Part model, mm, in its own coordinate system. A direction names the side the tool comes from. Give positions to 0.01 mm unless a question says otherwise; leave off trailing zeros. Write each loop counter-clockwise with the first axis right and the second up, starting at its lowest first coordinate (ties: lowest second). Pieces come first, ordered by that corner, then holes. Notation, with made-up numbers: (43.5, -14) - (99.5, -14) arc R8 ccw to (99.5, 0) - close; hole circle Ø5 at (37.25, 81.5). An arc over 180 degrees is marked (long way). Answer in a Markdown table with one row per item. Add a question column.
1. Probe line 1 along Y through (x, z) = (0, 1); line 2 along Y through (x, z) = (-20, 0.8); line 3 along X through (y, z) = (1, 4.75). List the from-to ranges inside material, lowest first.
2. Pull direction Y, two halves, no side cores. Call faces 6 (the flat face through (10, -30, 1)), 7 (the flat face through (-17.7, -2.3, 2)), 8 (the flat face through (-19, -8, 5)): released by +Y, released by -Y, zero draft, split by the parting line, or undercut.
3. Which spindle directions (+Z, -Z, +X, -X, +Y, -Y) get a long thin tool onto all of the face, cutting with end or side? Do faces 1 (the flat face through (18, -8, 5)), 2 (the flat face through (-20, -10, 1)), 3 (the flat face through (0, -48, 5)), 4 (the cylindrical face through (14.755, 0.231, 4.028)), 5 (the flat face through (-8, -28, 5)). Say none if no direction does.
4. Band-saw the part on A-A on x = 0. State how many separate pieces and enclosed holes the cut face has, plus the area to 3 significant figures.
5. Drop flat-ended pins along their axis: pin 1 Ø13.5 at (x, y) = (20, 0) entering from -Z; pin 2 Ø2.5 at (y, z) = (-21, 1.5) entering from +X; pin 3 Ø3.5 at (x, z) = (-23.5, 1) entering from -Y; pin 4 Ø6.5 at (x, y) = (0, 0) entering from +Z. Give the stop position or say it passes through.
6. Band-saw the part on D-D on x = 20. Write the cut outline in (y, z).
7. Band-saw the part on B-B on z = 5. Write the cut outline in (x, y).
```python
from build123d import *

# Parameters (mm, degrees)
F2_R     = 2.75
F3_DEPTH = 6
F4_SIZE  = 3
F5_R     = 5.25
F5_R_2   = 2.75
F6_DEPTH = 4


with BuildPart() as f3:
    # F2 (on Top) → F3 (new body)
    with BuildSketch(Plane.XY):
        Polygon((-10, -50), (0, -50), (10, -50), (10, -10), (30, -10), (30, 10), (0, 10), (-30, 10), (-30, -10), (-10, -10), align=None)
        with Locations((0, -40)):
            Circle(F2_R, mode=Mode.SUBTRACT)
        with Locations((-20, 0)):
            Circle(F2_R, mode=Mode.SUBTRACT)
        with Locations((0, -20)):
            Circle(F2_R, mode=Mode.SUBTRACT)
        Circle(F2_R, mode=Mode.SUBTRACT)
        with Locations((20, 0)):
            Circle(F2_R, mode=Mode.SUBTRACT)
    extrude(amount=F3_DEPTH)

    # F4
    f4_edges = [f3.edges().sort_by_distance(p)[0] for p in [
        (0, -50, 6),
        (10, -30, 6),
        (20, -10, 6),
        (30, 0, 6),
        (0, 10, 6),
        (-30, 0, 6),
        (-20, -10, 6),
        (-10, -30, 6),
    ]]
    chamfer(f4_edges, length=F4_SIZE)

    # F5 (on face) → F6 (cut)
    with BuildSketch(Plane.XY.offset(6)):
        with Locations((-20, 0)):
            Circle(F5_R)
        with Locations((-20, 0)):
            Circle(F5_R_2, mode=Mode.SUBTRACT)
        Circle(F5_R)
        Circle(F5_R_2, mode=Mode.SUBTRACT)
        with Locations((20, 0)):
            Circle(F5_R)
        with Locations((20, 0)):
            Circle(F5_R_2, mode=Mode.SUBTRACT)
        with Locations((0, -20)):
            Circle(F5_R)
        with Locations((0, -20)):
            Circle(F5_R_2, mode=Mode.SUBTRACT)
        with Locations((0, -40)):
            Circle(F5_R)
        with Locations((0, -40)):
            Circle(F5_R_2, mode=Mode.SUBTRACT)
    extrude(amount=-F6_DEPTH, mode=Mode.SUBTRACT)


solid = f3.part
```
Values:
| question | item | result |
|---|---|---|
| 1 | line 1 | y = -50 to -42.75, -37.25 to -22.75, -17.25 to -2.75, 2.75 to 10 |
| 1 | line 2 | y = -10 to -2.75, 2.75 to 10 |
| 1 | line 3 | x = -28.25 to -25.15, -14.85 to -5.15, 5.15 to 14.85, 25.15 to 28.25 |
| 2 | face 6 | zero draft |
| 2 | face 7 | undercut |
| 2 | face 8 | released by -Y |
| 3 | face 1 | +Z, +X, -Y |
| 3 | face 2 | +Z, -Z, -X, -Y |
| 3 | face 3 | +Z, +X, -X, -Y |
| 3 | face 4 | +Z |
| 3 | face 5 | +Z, -X, -Y |
| 4 | separate pieces | 4 |
| 4 | enclosed holes | 0 |
| 4 | area | 192 mm² |
| 5 | pin 1 | stops at z = 0 |
| 5 | pin 2 | stops at x = 10 |
| 5 | pin 3 | stops at y = -10 |
| 5 | pin 4 | stops at z = 2 |
| 6 | outline | (-10, 0) - (-2.75, 0) - (-2.75, 2) - (-5.25, 2) - (-5.25, 6) - (-7, 6) - (-10, 3) - close; (2.75, 0) - (10, 0) - (10, 3) - (7, 6) - (5.25, 6) - (5.25, 2) - (2.75, 2) - close |
| 7 | outline | (-28, -8) - (-8, -8) - (-8, -48) - (8, -48) - (8, -8) - (28, -8) - (28, 8) - (-28, 8) - close; hole circle Ø10.5 at (-20, 0); hole circle Ø10.5 at (0, -40); hole circle Ø10.5 at (0, -20); hole circle Ø10.5 at (0, 0); hole circle Ø10.5 at (20, 0) |
